Geometry: final body of the model. Coordinates: model frame, mm. Face numbers are marked on the shaded views. A direction names the side the tool comes from. Give positions to 0.01 mm unless a question says otherwise; leave off trailing zeros. Write each loop counter-clockwise with the first axis right and the second up, starting at its lowest first coordinate (ties: lowest second). Pieces come first, ordered by that corner, then holes. Notation, with made-up numbers: M 65.25,54 L 105.25,54 A20 ccw 105.25,69 Z; hole C 75.5,3.25 d7. An arc over 180 degrees is marked long. Use a Markdown table: item, result. Add a question column.
1) Set-up query: the marked faces 4 and 5. Return all of +Z, -Z, +X, -X, +Y, -Y with unobstructed straight access to the full face (end or side cutting, diameter ignored); none if empty.
2) Line query: line 1 (Y direction, x = 0.5, z = 1.2); line 2 (Z direction, x = 2.75, y = 5); line 3 (X direction, y = 0.25, z = 1.5). Output: solid intervals per line, ascending.
3) Draft query along X for the marked faces 1, 2 and 3. Return one class per face: +X half, -X half, draft (parallel to the pull), parting line (faces both ways), or undercut.
4) Pin query (flat end, axial travel): pin 1 (0.5 mm diameter, centred on x = 0.5, z = 1.5, fed in from +Y); pin 2 (1 mm diameter, centred on x = -4, y = -4.5, fed in from +Z); pin 3 (0.8 mm diameter, centred on y = 1.5, z = 1.5, fed in from +X). Return the tip coordinate at first contact, or that it passes through.
5) Section D-D on y = -3. Return the cut outline in (x, z), then the cut area to 3 significant figures.
6) Section A-A on z = 1.45. Return the cut outline in (x, y), then the cut area to 3 significant figures.
```python
from build123d import *

# Parameters (mm, degrees)
ESQUISSE1_W             = 12
ESQUISSE1_H             = 12.5
EXTRUSION1_DEPTH        = 1
EXTRUSION2_DEPTH        = 2
ENL_V_MAT_EXTRU_1_DEPTH = 2.25
CONG_1_R                = 0.02


with BuildPart() as part:
    # Esquisse1 → Extrusion1 (new body)
    with BuildSketch(Plane.XY):
        Rectangle(ESQUISSE1_W, ESQUISSE1_H)
    extrude(amount=EXTRUSION1_DEPTH)

    # Esquisse3 → Extrusion2 (add)
    with BuildSketch(Plane.XY):
        Polygon((-1.25, 2.9), (2.25, 2.9), (2.25, 0.65), (1.75, 0.15), (-1.25, 0.15), align=None)
    extrude(amount=EXTRUSION2_DEPTH)

    # Esquisse4 → Enlèv. mat.-Extru.1 (cut)
    with BuildSketch(Plane.XZ.offset(-0.4)):
        with BuildLine():
            Line((0.619431951, 2), (1.839642881, 2))
            ThreePointArc((1.839642881, 2), (1.229537416, 1.755105285), (0.619431951, 2))
        make_face()
        with BuildLine():
            Line((0.197380528, 2), (-1.022830402, 2))
            ThreePointArc((-1.022830402, 2), (-0.412724937, 1.755105285), (0.197380528, 2))
        make_face()
    extrude(amount=-ENL_V_MAT_EXTRU_1_DEPTH, mode=Mode.SUBTRACT)

    # Congé1
    cong_1_edges = [part.edges().sort_by_distance(p)[0] for p in [
        (0.5, 2.9, 2),
        (2.25, 1.775, 2),
        (2, 0.4, 2),
        (0.25, 0.15, 2),
        (-1.25, 1.525, 2),
        (1.229537416, 0.4, 2),
        (0.619431951, 1.525, 2),
        (1.229537416, 2.65, 2),
        (1.839642881, 1.525, 2),
        (-0.412724937, 0.4, 2),
        (-1.022830402, 1.525, 2),
        (-0.412724937, 2.65, 2),
        (0.197380528, 1.525, 2),
    ]]
    fillet(cong_1_edges, radius=CONG_1_R)


solid = part.part
```
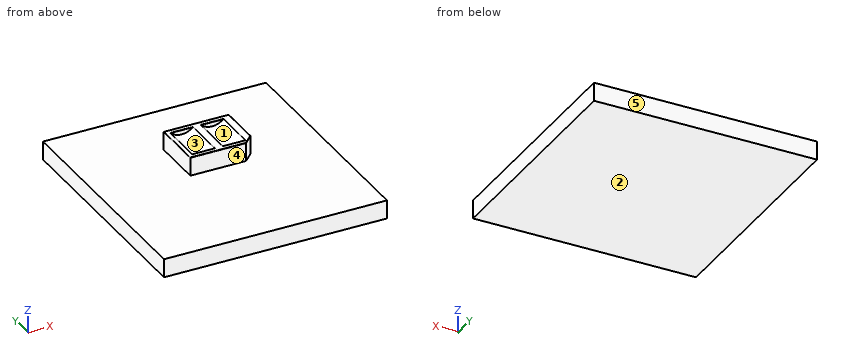
Found:
| question | item | result |
|---|---|---|
| 1 | face 4 | +Z, +X, -X, -Y |
| 1 | face 5 | +Z, -Z, +X, -X, +Y |
| 2 | line 1 | 0.15 to 2.9 |
| 2 | line 2 | 0 to 1 |
| 2 | line 3 | -1.25 to 1.85 |
| 3 | face 1 | undercut |
| 3 | face 2 | draft |
| 3 | face 3 | undercut |
| 4 | pin 1 | y = 2.9 |
| 4 | pin 2 | z = 1 |
| 4 | pin 3 | x = 2.25 |
| 5 | outline | M -6,0 L 6,0 L 6,1 L -6,1 Z |
| 5 | area | 12.0 mm² |
| 6 | outline | M -1.25,0.15 L 1.75,0.15 L 2.25,0.65 L 2.25,2.9 L -1.25,2.9 Z |
| 6 | area | 9.50 mm² |
